Geometry: final body of the model. Coordinates: model frame, mm. A direction names the side the tool comes from. Coordinates: 2 decimals unless noted, no trailing zeros. Order: outer loops, then holes, each group sorted by start corner. A loop starts at its lowest first (then second) coordinate and runs counter-clockwise, first axis right, second up. Notation, with made-up numbers: (16, -17) -> (23, -17) arc R15 ccw to (23, 9) -> close; hole circle Ø4 at (49, 66). An arc over 180 degrees is marked (long way). Use one line per item in the form item = value.
```python
from build123d import *

# Parameters (mm, degrees)
F0_W     = 549
F0_H     = 367.5
F1_DEPTH = 279
F2_T     = -7.5
F3_W     = 49.5
F3_H     = 367.5
F3_W_2   = 30
F4_DEPTH = 30


with BuildPart() as f1:
    # F0 (on Top) → F1 (new body)
    with BuildSketch(Plane.XY):
        with Locations((1.85414, -14.167297)):
            Rectangle(F0_W, F0_H)
    extrude(amount=F1_DEPTH)

    # F2
    f2_openings = [f1.faces().sort_by_distance(p)[0] for p in [
        (1.85414, -14.167297, 279),
        (1.85414, -14.167297, 0),
    ]]
    offset(amount=F2_T, openings=f2_openings)

    # F3 (on face) → F4 (join)
    with BuildSketch(Plane(origin=(0, 0, 0), x_dir=(1, 0, 0), z_dir=(0, 0, -1))):
        with Locations((-247.89586, 14.167297)):
            Rectangle(F3_W, F3_H)
        with Locations((1.85414, 14.167297)):
            Rectangle(F3_W_2, F3_H)
        with Locations((251.60414, 14.167297)):
            Rectangle(F3_W, F3_H)
    extrude(amount=F4_DEPTH)


solid = f1.part
```
1) Pull-direction query (Y, two-part tool) for faces 1 (the flat face through (248, -17, 0)), 2 (the flat face through (-13.146, -12, -15)), 3 (the flat face through (-2, -190.417, 138)), 4 (the flat face through (-2, -197.917, 127)); classes: released by +Y, released by -Y, zero draft, split by the parting line, or undercut.
Results found:
face_1 = undercut
face_2 = zero draft
face_3 = undercut
face_4 = released by -Y
2) Contact query for flat-ended pins moving along their axis: P1, Ø4, axis at x = -149.5, y = 164.5, coming from the -Z side; P2, Ø4, axis at x = 18.5, y = -137, coming from the +Z side. Output: stop coordinate, or through.
Results found:
P1 = 0
P2 = 0
3) Section B-B, the plane y = 11.5. Output: boundary loops of the cut face in (x, z).
Results found:
outline = (-272.65, -30) -> (-223.15, -30) -> (-223.15, 0) -> (-265.15, 0) -> (-265.15, 279) -> (-272.65, 279) -> close; (-13.15, -30) -> (16.85, -30) -> (16.85, 0) -> (-13.15, 0) -> close; (226.85, -30) -> (276.35, -30) -> (276.35, 279) -> (268.85, 279) -> (268.85, 0) -> (226.85, 0) -> close
4) Material intervals for probe 1 along X at (y, z) = (22, 94); probe 2 along X at (y, z) = (155, -14); probe 3 along Y at (x, z) = (-149, 140.5), sorted ascending. Write a range as from..to.
Results found:
probe_1 = -272.65..-265.15, 268.85..276.35
probe_2 = -272.65..-223.15, -13.15..16.85, 226.85..276.35
probe_3 = -197.92..-190.42, 162.08..169.58
5) Access query for faces 5 (the flat face through (251, -17, -30)), 6 (the flat face through (-244, -17, 0)). Directions: +Z, -Z, +X, -X, +Y, -Y. A direction counts if a zero-diameter tool reaches every point of the face in a straight line with its end or side. Return the directions, or none.
Results found:
face_5 = -Z, +X, -X, +Y, -Y
face_6 = +Z
6) Section C-C, the plane z = 44.5. Output: boundary loops of the cut face in (x, y).
Results found:
outline = (-272.65, -197.92) -> (276.35, -197.92) -> (276.35, 169.58) -> (-272.65, 169.58) -> close; hole (-265.15, -190.42) -> (268.85, -190.42) -> (268.85, 162.08) -> (-265.15, 162.08) -> close
7) Section A-A, the plane x = -98.5. Output: boundary loops of the cut face in (y, z), and give its area (4 significant figures).
Results found:
outline = (-197.92, 0) -> (-190.42, 0) -> (-190.42, 279) -> (-197.92, 279) -> close; (162.08, 0) -> (169.58, 0) -> (169.58, 279) -> (162.08, 279) -> close
area = 4,185 mm2
